Check sheet for the modelled part. Datum: model origin and axes. Units: mm. A direction names the side the tool comes from. Round coordinates to 2 decimals unless told otherwise and drop trailing zeros. Order: outer loops, then holes, each group sorted by start corner. A loop starts at its lowest first (then second) coordinate and runs counter-clockwise, first axis right, second up.
from build123d import *

# Parameters (mm, degrees)
EXTRUDE_1_DEPTH      = 15
EXTRUDE_1_DEPTH_BACK = 15
EXTRUDE_2_DEPTH      = 8
SKETCH_3_W           = 10.666666667
SKETCH_3_H           = 14
CUT_EXTRUDE_1_DEPTH  = 43.766809561


with BuildPart() as part:
    # Эскиз1 → Бобышка-Вытянуть1 (new, two sides: drawn at the far end of the back side and taken through both)
    with BuildSketch(Plane.XY.offset(-EXTRUDE_1_DEPTH_BACK)):
        Polygon((-6.666666667, -5), (-20, -5), (-20, -15), (20, -15), (20, 15), (-6.666666667, 15), align=None)
    extrude(amount=EXTRUDE_1_DEPTH + EXTRUDE_1_DEPTH_BACK)

    # Эскиз2 → Бобышка-Вытянуть2 (add)
    with BuildSketch(Plane.XY.offset(15)):
        Polygon((-20, -15), (20, 15), (20, -15), align=None)
    extrude_2 = extrude(amount=EXTRUDE_2_DEPTH)

    # Зеркальное отражение1: Бобышка-Вытянуть2 across plane
    add(extrude_2.mirror(Plane.XY))

    # Эскиз3 → Вырез-Вытянуть1 (cut, through all)
    with BuildSketch(Plane(origin=(0, 15, 0), x_dir=(1, 0, 0), z_dir=(0, 1, 0))):
        with Locations((6.666666667, 0)):
            Rectangle(SKETCH_3_W, SKETCH_3_H)
    extrude(amount=-CUT_EXTRUDE_1_DEPTH, mode=Mode.SUBTRACT)


solid = part.part
1) Gauge pin test, flat ends, axial feed: pin 1 (1.5 mm diameter, centred on y = 4, z = 10.5, fed in from -X); pin 2 (4 mm diameter, centred on x = 11, z = -1, fed in from +Y); pin 3 (10.5 mm diameter, centred on x = -14.5, z = 7.5, fed in from +Y); pin 4 (8 mm diameter, centred on x = 7, z = 1.5, fed in from +Y). Record the tip position at first contact, or that the pin passes through.
2) Draft check along X on faces 6 (the face through (20, 0, 0)), 7 (the face through (9, -6, 23)), 8 (the face through (1.333, 0, 0)). Enter one of: pulls with the +X half, pulls with the -X half, needs draft (parallel to the pull), parting line crosses it, or undercut.
3) Sectioned sample at B-B on x = -13. Record the cut outline in (y, z).
4) Set-up check for faces 1 (the face through (4, 7, -15)), 2 (the face through (7, 0, -7)), 3 (the face through (-15, -9, 15)), 4 (the face through (-6.667, 5, 0)), 5 (the face through (1, 15, 0)): record each of +Z, -Z, +X, -X, +Y, -Y from which the full face is reachable in a straight line by a thin tool's end or side.
5) Sectioned sample at A-A on z = 4.5. Record the cut outline in (x, y), and give its area (3 significant figures).
6) Sectioned sample at D-D on z = -10. Record the cut outline in (x, y).
7) Scan lines: line 1 (X direction, y = 13.5, z = -2.5); line 2 (Z direction, x = 5, y = -9); line 3 (X direction, y = -1, z = 10). Record each from-to range of solid material in increasing order.
8) Sectioned sample at C-C on y = 10.5. Record the cut outline in (x, z), and give its area (3 significant figures).
Values found:
1. pin 1: stops at x = -6.67
1. pin 2: stops at y = 15
1. pin 3: stops at y = -5
1. pin 4: passes through
2. face 6: pulls with the +X half
2. face 7: needs draft
2. face 8: undercut
3. outline: (-15, -23) - (-9.75, -23) - (-9.75, -15) - (-5, -15) - (-5, 15) - (-9.75, 15) - (-9.75, 23) - (-15, 23) - close
4. face 1: -Z, -X, +Y
4. face 2: +Y, -Y
4. face 3: +Z, -X, +Y
4. face 4: +Z, -Z, -X, +Y
4. face 5: +Z, -Z, +X, -X, +Y
5. outline: (-20, -15) - (1.33, -15) - (1.33, 15) - (-6.67, 15) - (-6.67, -5) - (-20, -5) - close; (12, -15) - (20, -15) - (20, 15) - (12, 15) - close
5. area: 613 mm2
6. outline: (-20, -15) - (20, -15) - (20, 15) - (-6.67, 15) - (-6.67, -5) - (-20, -5) - close
7. line 1: x = -6.67 to 1.33, 12 to 20
7. line 2: z = -23 to -7, 7 to 23
7. line 3: x = -6.67 to 20
8. outline: (-6.67, -15) - (14, -15) - (14, -23) - (20, -23) - (20, 23) - (14, 23) - (14, 15) - (-6.67, 15) - close; hole (1.33, -7) - (12, -7) - (12, 7) - (1.33, 7) - close
8. area: 747 mm2
